For this review, use the dimensioned drawing (mm, ordinates from the lowest corner) and the shaded views. A direction names the side the tool comes from. Give positions to 0.01 mm unless a question says otherwise; leave off trailing zeros. Loops run counter-clockwise (first coordinate to the right, second up) from the corner with the lowest first, then second, coordinate; pieces in that order, holes last. Notation, with made-up numbers: M 36.5,-30.75 L 95.5,-30.75 A20 cw 95.5,-15.75 Z; hole C -31,35 d11. An arc over 180 degrees is marked long. Use CSV: the item, a comma, the result in double quotes.
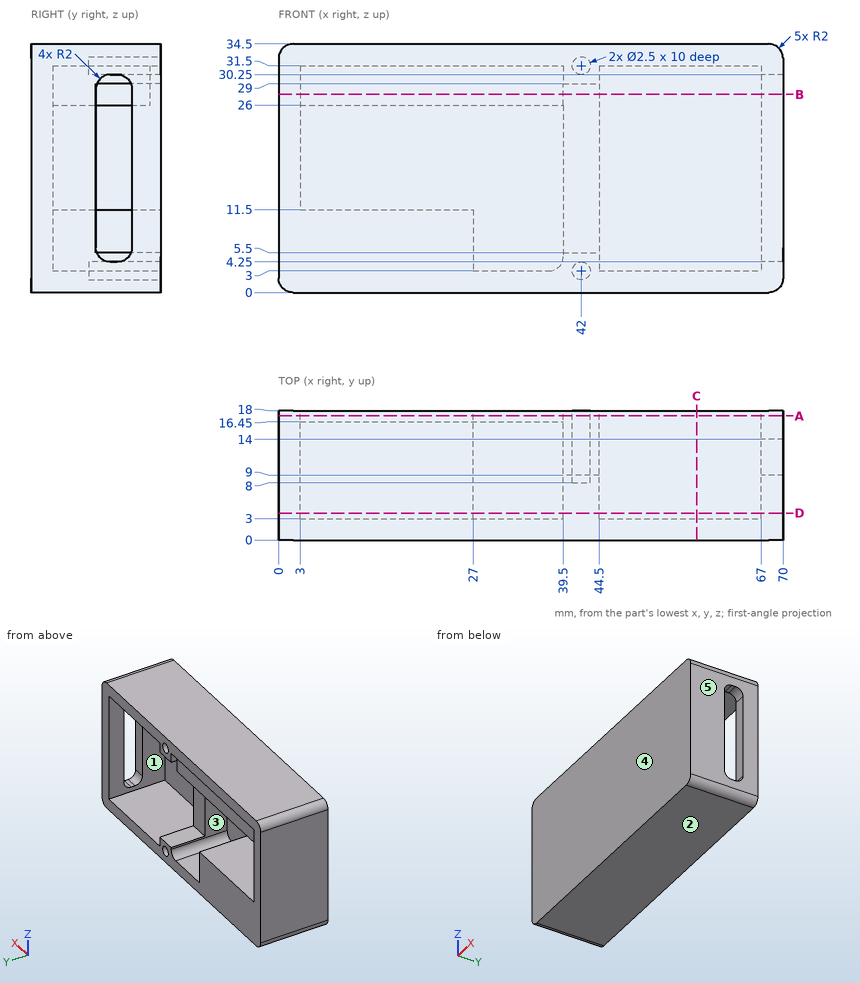
(1) We need section A-A on y = 17.25. State the section outline as (x, z) points.
A:
outline,"M 0,2 A2 ccw 2,0 L 68,0 A2 ccw 70,2 L 70,32.5 A2 ccw 68,34.5 L 2,34.5 A2 ccw 0,32.5 Z; hole M 3,11.5 L 27,11.5 L 27,3 L 37.5,3 A2 ccw 39.5,5 L 39.5,5.5 L 44.5,5.5 L 44.5,3 L 67,3 L 67,31.5 L 44.5,31.5 L 44.5,29 L 39.5,29 L 39.5,31.5 L 3,31.5 Z; hole C 42,3 d2.5; hole C 42,31.5 d2.5"
(2) We need section C-C on x = 58. State the section outline as (y, z) points, then the cut area to 4 significant figures.
A:
outline,"M 0,0 L 18,0 L 18,3 L 3,3 L 3,31.5 L 18,31.5 L 18,34.5 L 0,34.5 Z"
area,"193.5 mm²"
(3) Machinability: for the marked faces 1 and 2, which of the approach directions +Z, -Z, +X, -X, +Y, -Y give a long, thin tool a straight path to every point of the face, cutting with its end or side? Answer none if there is none.
A:
face 1,"+Y"
face 2,"-Z, +X, -X, +Y, -Y"
(4) Wall thickness on line 1 along X through (y, z) = (14.75, 5); line 2 along X through (y, z) = (6, 24); line 3 along Z through (x, y) = (41.5, 14.75): over which ranges is each line inside the solid? List them lowest first. Write a range as [from, to].
A:
line 1,"[0, 27], [39.5, 44.5], [67, 70]"
line 2,"[0, 3], [39.5, 44.5], [67, 70]"
line 3,"[0, 1.85], [4.15, 5.5], [29, 30.35], [32.65, 34.5]"
(5) Clearance check with flat-ended pins moving along their axes: P1, Ø7, axis at x = 56, z = 19, coming from the +Y side; P2, Ø4, axis at x = 41.5, z = 14.5, coming from the +Y side; P3, Ø0.5, axis at x = 69, y = 11.5, coming from the +Z side. State where each tip first meets the part, or that it passes through.
A:
P1,"y = 3"
P2,"y = 9"
P3,"z = 34.35"
(6) We need section D-D on y = 3.75. State the section outline as (x, z) points, then the cut area to 3 significant figures.
A:
outline,"M 0,2 A2 ccw 2,0 L 68,0 A2 ccw 70,2 L 70,32.5 A2 ccw 68,34.5 L 2,34.5 A2 ccw 0,32.5 Z; hole M 3,11.5 L 27,11.5 L 27,3 L 37.5,3 A2 ccw 39.5,5 L 39.5,26 L 3,26 Z; hole M 44.5,3 L 67,3 L 67,31.5 L 44.5,31.5 Z"
area,"1,140 mm²"
(7) The part is to be moulded in two halves that separate along X. For the marked faces 3, 4 and 5, say which applies: released by +X, released by -X, zero draft, split by the parting line, or undercut.
A:
face 3,"undercut"
face 4,"zero draft"
face 5,"released by +X"
(8) We need section B-B on z = 27.5. State the section outline as (x, y) points, then the cut area to 3 significant figures.
A:
outline,"M 0,0 L 70,0 L 70,9 L 67,9 L 67,3 L 44.5,3 L 44.5,9 L 39.5,9 L 39.5,16.45 L 3,16.45 L 3,18 L 0,18 Z; M 67,14 L 70,14 L 70,18 L 67,18 Z"
area,"806 mm²"
